from build123d import *

# Parameters (mm, degrees)
F0_W     = 32.5
F0_H     = 17.5
F0_R     = 1.25
F1_DEPTH = 1.5
F2_W     = 16.95
F2_H     = 10.8
F2_W_2   = 14.55
F2_H_2   = 8.4
F3_DEPTH = 12.25
F4_W     = 9.15
F4_H     = 10.5
F5_DEPTH = 1.2
F6_W     = 6
F6_H     = 8.5
F7_DEPTH = 1.2
F8_W     = 12.55
F8_H     = 6.4
F9_DEPTH = 25


with BuildPart() as f1:
    # F0 (on Top) → F1 (new body)
    with BuildSketch(Plane.XY):
        Rectangle(F0_W, F0_H)
        with Locations((-14, 0)):
            Circle(F0_R, mode=Mode.SUBTRACT)
        with Locations((14, 0)):
            Circle(F0_R, mode=Mode.SUBTRACT)
    extrude(amount=F1_DEPTH)

    # F2 (on face) → F3 (join)
    with BuildSketch(Plane.XY.offset(1.5)):
        Rectangle(F2_W, F2_H)
        Rectangle(F2_W_2, F2_H_2, mode=Mode.SUBTRACT)
    extrude(amount=F3_DEPTH)

    # F4 (on face) → F5 (cut, through all)
    with BuildSketch(Plane.XZ.offset(5.4)):
        with Locations((0.4, 8.5)):
            Rectangle(F4_W, F4_H)
    extrude(amount=-F5_DEPTH, mode=Mode.SUBTRACT)

    # F6 (on face) → F7 (cut, through all)
    with BuildSketch(Plane(origin=(0, 5.4, 0), x_dir=(-1, 0, 0), z_dir=(0, 1, 0))):
        with Locations((4.275, 5.75)):
            Rectangle(F6_W, F6_H)
    extrude(amount=-F7_DEPTH, mode=Mode.SUBTRACT)

    # F8 (on face) → F9 (cut)
    with BuildSketch(Plane.XY.offset(1.5)):
        Rectangle(F8_W, F8_H)
    extrude(amount=-F9_DEPTH, mode=Mode.SUBTRACT)


solid = f1.part
Design review of the part built by this model. Coordinates are the model's own, in mm. A direction names the side the tool comes from. Round coordinates to 2 decimals unless told otherwise and drop trailing zeros. Write each loop counter-clockwise with the first axis right and the second up, starting at its lowest first coordinate (ties: lowest second). Pieces come first, ordered by that corner, then holes.
Item 1: Consider section C-C on z = 3.75. Give the boundary of the cut face in (x, y) (3 decimals), and give its area (3 significant figures).
Item 2: Consider section B-B on y = -2. Give the boundary of the cut face in (x, z) (3 decimals).
Item 3: For pin 1 Ø3 at (y, z) = (-1, 7.5) entering from +X (3 decimals); pin 2 Ø1.3 at (y, z) = (5, 5.5) entering from -X (3 decimals); pin 3 Ø3 at (x, y) = (12, -4) entering from +Z; pin 4 Ø1.5 at (x, y) = (-14, 0) entering from -Z, all flat-tipped, find the tip position at first contact; note any pin that passes through.
Item 4: Draft analysis for pull direction Y (two halves, no side actions). For faces 6 (the flat face through (-6.275, 0, 1)), 7 (the flat face through (4.975, -5, 8)), 8 (the flat face through (2, 5.4, 8)), state which applies: released by +Y, released by -Y, zero draft, split by the parting line, or undercut.
Item 5: For faces 1 (the flat face through (6.275, 0, 1)), 2 (the flat face through (7.275, 0, 8)), 3 (the flat face through (0, -5, 3.25)), 4 (the flat face through (-4, 5, 10)), 5 (the flat face through (0, -8.75, 1)), list the 3-axis set-ups (+Z, -Z, +X, -X, +Y, -Y) from which the entire face can be reached by the end or side of a thin tool; tool diameter is ignored.
Item 6: Consider section A-A on x = 14. Give the boundary of the cut face in (y, z), and give its area (3 significant figures).
Item 7: Consider section D-D on y = 0. Give the boundary of the cut face in (x, z) (3 decimals).
Item 8: Wall thickness on L1, parallel to Y at x = -14, z = 0.55; L2, parallel to X at y = 3.5, z = 8 (3 decimals); L3, parallel to Z at x = 2.5, y = -4.5: over which ranges is each line inside the solid? List them lowest first.
Check values:
1. outline: (-8.475, -5.4) - (-4.175, -5.4) - (-4.175, -4.2) - (-7.275, -4.2) - (-7.275, 5.4) - (-8.475, 5.4) - close; (-1.275, 4.2) - (7.275, 4.2) - (7.275, -4.2) - (4.975, -4.2) - (4.975, -5.4) - (8.475, -5.4) - (8.475, 5.4) - (-1.275, 5.4) - close
1. area: 42.7 mm2
2. outline: (-16.25, 0) - (-6.275, 0) - (-6.275, 1.5) - (-7.275, 1.5) - (-7.275, 13.75) - (-8.475, 13.75) - (-8.475, 1.5) - (-16.25, 1.5) - close; (6.275, 0) - (16.25, 0) - (16.25, 1.5) - (8.475, 1.5) - (8.475, 13.75) - (7.275, 13.75) - (7.275, 1.5) - (6.275, 1.5) - close
3. pin 1: stops at x = 8.475
3. pin 2: stops at x = -8.475
3. pin 3: stops at z = 1.5
3. pin 4: passes through
4. face 6: undercut
4. face 7: zero draft
4. face 8: released by +Y
5. face 1: +Z, -Z
5. face 2: +Z
5. face 3: +Z, -Y
5. face 4: +Y
5. face 5: +Z, -Z, +X, -X, -Y
6. outline: (-8.75, 0) - (-1.25, 0) - (-1.25, 1.5) - (-8.75, 1.5) - close; (1.25, 0) - (8.75, 0) - (8.75, 1.5) - (1.25, 1.5) - close
6. area: 22.5 mm2
7. outline: (-16.25, 0) - (-15.25, 0) - (-15.25, 1.5) - (-16.25, 1.5) - close; (-12.75, 0) - (-6.275, 0) - (-6.275, 1.5) - (-7.275, 1.5) - (-7.275, 13.75) - (-8.475, 13.75) - (-8.475, 1.5) - (-12.75, 1.5) - close; (6.275, 0) - (12.75, 0) - (12.75, 1.5) - (8.475, 1.5) - (8.475, 13.75) - (7.275, 13.75) - (7.275, 1.5) - (6.275, 1.5) - close; (15.25, 0) - (16.25, 0) - (16.25, 1.5) - (15.25, 1.5) - close
8. L1: y = -8.75 to -1.25, 1.25 to 8.75
8. L2: x = -8.475 to -7.275, 7.275 to 8.475
8. L3: z = 0 to 3.25
